CAD build for the part. Positions are in the model's coordinates, mm. A direction names the side the tool comes from. Round coordinates to 2 decimals unless told otherwise and drop trailing zeros. Write each loop counter-clockwise with the first axis right and the second up, starting at its lowest first coordinate (ties: lowest second). Pieces come first, ordered by that corner, then holes. Notation, with made-up numbers: (45, -17.5) -> (95, -17.5) arc R13 ccw to (95, 6.5) -> close; hole circle Ø4 at (13.5, 24). An arc over 180 degrees is marked (long way). Put each result on its own line as item: value. Start each with the question number.
1. Saw through at C-C on z = 7.5. List the corners of the cut face in (x, y).
2. Saw through at D-D on z = 0. List the corners of the cut face in (x, y).
3. Saw through at B-B on x = 0. List the corners of the cut face in (y, z), and give its area (3 significant figures).
4. 3-axis set-ups, long thin cutter, end or side, ignore diameter. For faces 1 (the cylindrical face through (4.24, 5.47, -6.23)), 2 (the flat face through (-3.5, 5, 0)), 3 (the cylindrical face through (-4.26, 5.59, -8.07)): which of +Z, -Z, +X, -X, +Y, -Y reach the whole face in a straight line?
5. Drill centre lines: line 1 (Z direction, x = 4.75, y = 4.5); line 2 (Z direction, x = -4.1, y = 4.5); line 3 (Y direction, x = -4, z = 7.5). Where is each one in solid material? Low to high. Write a range as from..to.
6. Flat gauge pin, fed straight in: P1, Ø2, axis at x = 0, z = -1.5, coming from the +Y side. Where does the tip first touch, or does it go through?
7. Pull direction Z, two halves, no side cores. Call faces 4 (the cylindrical face through (0.748, 0.74, -0.976)), 5 (the flat face through (0, 1, 12.5)), 6 (the flat face through (0, 1, -12.5)), 7 (the flat face through (-4, 8, 0)): pulls with the +Z half, pulls with the -Z half, needs draft (parallel to the pull), parting line crosses it, or undercut.
8. Saw through at A-A on y = 7. List the corners of the cut face in (x, z), and give its area (3 significant figures).
Autodesk Inventor part; units mm, degrees
ref_plane "YZ Plane" through (0, 0, 0) normal (1, 0, 0) x (0, 1, 0)
ref_plane "XZ Plane" through (0, 0, 0) normal (0, 1, 0) x (-1, 0, 0)
ref_plane "XY Plane" through (0, 0, 0) normal (0, 0, 1) x (1, 0, 0)
sketch "Náčrt1" plane through (0, 0, 0) normal (0, 0, 1) x (1, 0, 0)
  line L0 (-5, 8) -> (-5, 0)
  line L1 (-5, 0) -> (5, 0)
  line L2 (5, 0) -> (5, 8)
  line L3 (5, 8) -> (3.5, 8)
  line L4 (3.5, 8) -> (3.5, 1.5)
  line L5 (3.5, 1.5) -> (-3.5, 1.5)
  line L6 (-3.5, 1.5) -> (-3.5, 8)
  line L7 (-3.5, 8) -> (-5, 8)
  line L8 (-7, 0) -> (7, 0)
  line L9 (0, 9.6) -> (0, -1.6)
  point P0 (0, 0)
  dimension "d0" = 8
  dimension "d1" = 10
  dimension "d2" = 1.5
  dimension "d3" = 1.5
  dimension "d4" = 1.5
extrude "Vysunutí1" add sketch "Náčrt1" along normal mid plane 25
sketch "Náčrt2" plane through (5, 0, 12.5) normal (1, 0, 0) x (0, 0, -1)
  line L0 (25, 8) -> (25, 0)
  line L1 (0, 0) -> (0, 8)
  line L2 (25, 8) -> (0, 8)
  point P0 (12.5, 0)
  point P1 (5, 4.5)
  point P2 (20, 4.5)
  dimension "d7" = 5
  dimension "d8" = 5
  dimension "d9" = 3.5
  dimension "d10" = 3.5
hole "Díra1" at (5, 4.5, 7.5) at (5, 4.5, -7.5) direction (-1, 0, 0) diameter 2.459 end through all counterbore diameter 3.2 counterbore depth 2
sketch "Náčrt3" plane through (-3.5, 1.5, 12.5) normal (0, 1, 0) x (1, 0, 0)
  line L0 (0, 25) -> (0, 0)
  point P0 (3.5, 12.5)
  point P1 (3.5, 12.5)
hole "Díra2" at (0, 1.5, 0) direction (0, -1, 0) diameter 2.459 end through all
properties part number "x_belt_anchor" material "Hliník 6061"
Return value:
1. outline: (-5, 0) -> (5, 0) -> (5, 2.9) -> (3.5, 2.9) -> (3.5, 1.5) -> (-3.5, 1.5) -> (-3.5, 3.27) -> (-5, 3.27) -> close; (-5, 5.73) -> (-3.5, 5.73) -> (-3.5, 8) -> (-5, 8) -> close; (3.5, 6.1) -> (5, 6.1) -> (5, 8) -> (3.5, 8) -> close
2. outline: (-5, 0) -> (-1.23, 0) -> (-1.23, 1.5) -> (-3.5, 1.5) -> (-3.5, 8) -> (-5, 8) -> close; (1.23, 0) -> (5, 0) -> (5, 8) -> (3.5, 8) -> (3.5, 1.5) -> (1.23, 1.5) -> close
3. outline: (0, -12.5) -> (1.5, -12.5) -> (1.5, -1.23) -> (0, -1.23) -> close; (0, 1.23) -> (1.5, 1.23) -> (1.5, 12.5) -> (0, 12.5) -> close
3. area: 33.8 mm^2
4. face 1: +X
4. face 2: +Z, -Z, +Y
4. face 3: +X, -X
5. line 1: z = -12.5..-9.1, -5.9..5.9, 9.1..12.5
5. line 2: z = -12.5..-8.73, -6.27..6.27, 8.73..12.5
5. line 3: y = 0..3.27, 5.73..8
6. P1: stops at y = 1.5
7. face 4: undercut
7. face 5: pulls with the +Z half
7. face 6: pulls with the -Z half
7. face 7: needs draft
8. outline: (-5, -12.5) -> (-3.5, -12.5) -> (-3.5, 12.5) -> (-5, 12.5) -> close; (3.5, -12.5) -> (5, -12.5) -> (5, 12.5) -> (3.5, 12.5) -> close
8. area: 75.0 mm^2
